Could you check a few things on this drawing? It's one solid part, dimensions in mm from its lowest x, y, z. A direction names the side the tool comes from. Give positions to 0.01 mm unless a question says otherwise; leave off trailing zeros. Order: outer loops, then holes, each group sorted by start corner. A loop starts at its lowest first (then second) coordinate and runs counter-clockwise, first axis right, second up. Notation, with made-up numbers: (82.5, 30.25) - (115.5, 30.25) arc R13 ccw to (115.5, 50.25) - close; hole circle Ø11 at (37.5, 72). An arc over 180 degrees is marked (long way). Return JSON: item names as keys, results as strings.
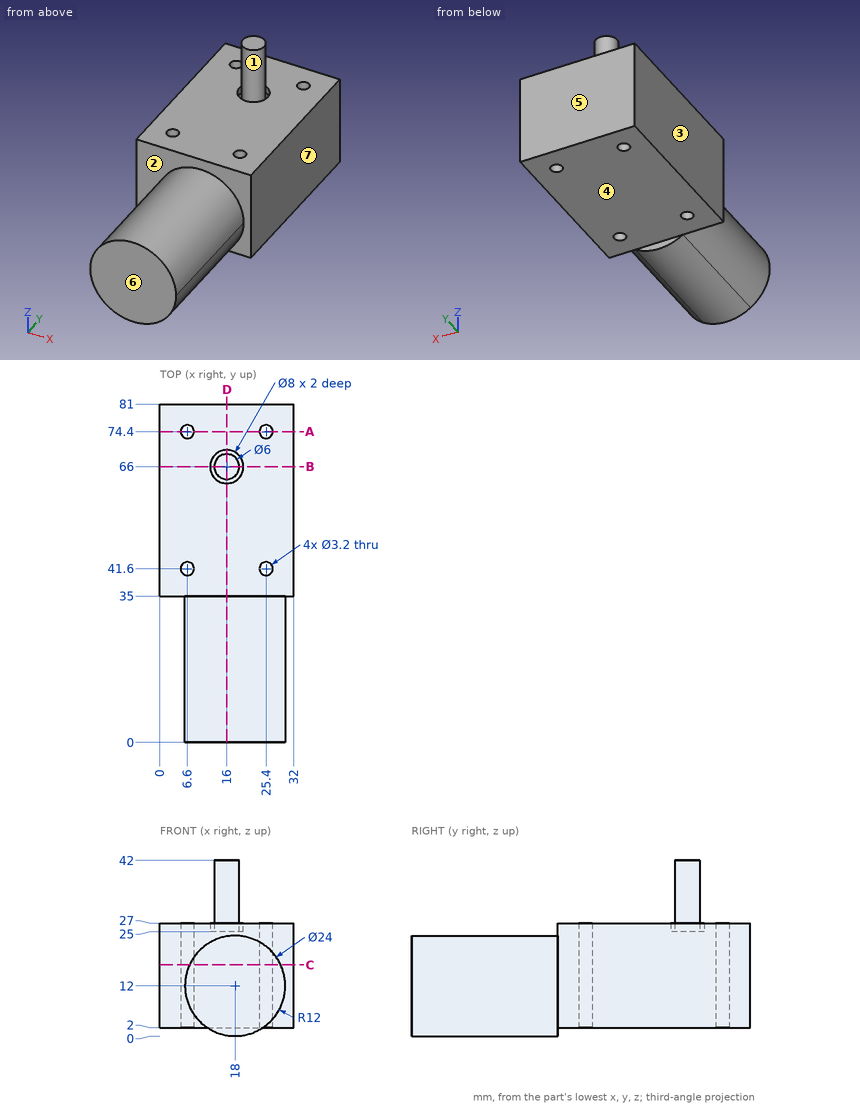
1. Suppose I cut it at B-B (y = 66). List the corners of the cut face in (x, z) for me, plus the area to 3 significant figures.
Checks:
{"outline": "(0, 2) - (32, 2) - (32, 27) - (20, 27) - (20, 25) - (19, 25) - (19, 42) - (13, 42) - (13, 25) - (12, 25) - (12, 27) - (0, 27) - close", "area": "886 mm^2"}
2. Suppose I cut it at D-D (x = 16). List the corners of the cut face in (y, z) for me, plus the area to 3 significant figures.
Checks:
{"outline": "(0, 0.17) - (35, 0.17) - (35, 2) - (81, 2) - (81, 27) - (70, 27) - (70, 25) - (69, 25) - (69, 42) - (63, 42) - (63, 25) - (62, 25) - (62, 27) - (35, 27) - (35, 23.83) - (0, 23.83) - close", "area": "2,060 mm^2"}
3. Suppose I cut it at C-C (z = 17). List the corners of the cut face in (x, y) for me.
Checks:
{"outline": "(0, 35) - (7.09, 35) - (7.09, 0) - (28.91, 0) - (28.91, 35) - (32, 35) - (32, 81) - (0, 81) - close; hole circle Ø3.2 at (6.6, 41.6); hole circle Ø3.2 at (6.6, 74.4); hole circle Ø3.2 at (25.4, 41.6); hole circle Ø3.2 at (25.4, 74.4)"}
4. On a 3-axis mill with a long thin cutter (end or side, diameter ignored), from which of +Z, -Z, +X, -X, +Y, -Y can I reach the whole of each face in a straight line? I mean the marked faces 1, 2, 3 and 4. Say none if no direction works.
Checks:
{"face 1": "+Z", "face 2": "-Y", "face 3": "+Z, -Z, -X, +Y, -Y", "face 4": "-Z, +X, -X, +Y"}
5. For pin 1 Ø10 at (x, y) = (7, 66) entering from -Z; pin 2 Ø5 at (x, y) = (6.6, 41.6) entering from +Z; pin 3 Ø1.9 at (x, y) = (25.4, 74.4) entering from -Z; pin 4 Ø4 at (x, z) = (17.5, 34.5) entering from -Y, each with a flat end and sliding along its axis, tell me the tip position at first contact or that it passes through.
Checks:
{"pin 1": "z = 2", "pin 2": "z = 27", "pin 3": "through", "pin 4": "y = 63"}
6. Suppose I cut it at A-A (y = 74.4). List the corners of the cut face in (x, z) for me.
Checks:
{"outline": "(0, 2) - (5, 2) - (5, 27) - (0, 27) - close; (8.2, 2) - (23.8, 2) - (23.8, 27) - (8.2, 27) - close; (27, 2) - (32, 2) - (32, 27) - (27, 27) - close"}
7. If I drill on L1, parallel to Y at x = 6.6, z = 17.5; L2, parallel to X at y = 74.4, z = 15.25; L3, parallel to Y at x = 25.4, z = 10.25, over which ranges is the centre line in solid material (lowest first)? Write a range as [from, to].
Checks:
{"L1": "[35, 40], [43.2, 72.8], [76, 81]", "L2": "[0, 5], [8.2, 23.8], [27, 32]", "L3": "[0, 40], [43.2, 72.8], [76, 81]"}
8. Thinking about a two-plate mould opening in Y: for the marked faces 5, 6 and 7, which applies, +Y half, -Y half, draft (parallel to the pull), parting line (faces both ways), or undercut?
Checks:
{"face 5": "+Y half", "face 6": "-Y half", "face 7": "draft"}
